from build123d import *

# Parameters (mm, degrees)
SKETCH1_R           = 2.2
SKETCH1_R_2         = 1.7
BOSS_EXTRUDE1_DEPTH = 6


with BuildPart() as part:
    # Sketch1 → Boss-Extrude1 (new body)
    with BuildSketch(Plane.XY.offset(3)):
        with BuildLine():
            Line((40.555136163, -29), (40.555136163, 17))
            ThreePointArc((40.555136163, 17), (42.019602257, 20.535533906), (45.555136163, 22))
            Line((45.555136163, 22), (54, 22))
            Line((54, 22), (74, 42))
            Line((74, 42), (74, 64))
            ThreePointArc((74, 64), (72.828427125, 66.828427125), (70, 68))
            Line((70, 68), (69, 68))
            ThreePointArc((69, 68), (68.292893219, 68.292893219), (68, 69))
            Line((68, 69), (68, 100))
            Line((68, 100), (56.5, 100))
            Line((56.5, 100), (56.5, 62.4))
            ThreePointArc((56.5, 62.4), (55.035533906, 58.864466094), (51.5, 57.4))
            Line((51.5, 57.4), (46.5, 57.4))
            ThreePointArc((46.5, 57.4), (42.964466094, 58.864466094), (41.5, 62.4))
            Line((41.5, 62.4), (41.5, 100))
            Line((41.5, 100), (-41.5, 100))
            Line((-41.5, 100), (-41.5, 62.4))
            ThreePointArc((-41.5, 62.4), (-42.964466094, 58.864466094), (-46.5, 57.4))
            Line((-46.5, 57.4), (-51.5, 57.4))
            ThreePointArc((-51.5, 57.4), (-55.035533906, 58.864466094), (-56.5, 62.4))
            Line((-56.5, 62.4), (-56.5, 100))
            Line((-56.5, 100), (-68, 100))
            Line((-68, 100), (-68, 69))
            ThreePointArc((-68, 69), (-68.292893219, 68.292893219), (-69, 68))
            Line((-69, 68), (-70, 68))
            ThreePointArc((-70, 68), (-72.828427125, 66.828427125), (-74, 64))
            Line((-74, 64), (-74, 42))
            Line((-74, 42), (-54, 22))
            Line((-54, 22), (-45.555136163, 22))
            ThreePointArc((-45.555136163, 22), (-42.019602257, 20.535533906), (-40.555136163, 17))
            Line((-40.555136163, 17), (-40.555136163, -29))
            ThreePointArc((-40.555136163, -29), (-42.019602257, -32.535533906), (-45.555136163, -34))
            Line((-45.555136163, -34), (-66, -34))
            Line((-66, -34), (-74, -42))
            Line((-74, -42), (-74, -64))
            ThreePointArc((-74, -64), (-72.828427125, -66.828427125), (-70, -68))
            Line((-70, -68), (-69, -68))
            ThreePointArc((-69, -68), (-68.292893219, -68.292893219), (-68, -69))
            Line((-68, -69), (-68, -100))
            Line((-68, -100), (-56.5, -100))
            Line((-56.5, -100), (-56.5, -61.8))
            ThreePointArc((-56.5, -61.8), (-55.035533906, -58.264466094), (-51.5, -56.8))
            Line((-51.5, -56.8), (-25.5, -56.8))
            ThreePointArc((-25.5, -56.8), (-21.964466094, -58.264466094), (-20.5, -61.8))
            Line((-20.5, -61.8), (-20.5, -100))
            Line((-20.5, -100), (20.5, -100))
            Line((20.5, -100), (20.5, -61.8))
            ThreePointArc((20.5, -61.8), (21.964466094, -58.264466094), (25.5, -56.8))
            Line((25.5, -56.8), (51.5, -56.8))
            ThreePointArc((51.5, -56.8), (55.035533906, -58.264466094), (56.5, -61.8))
            Line((56.5, -61.8), (56.5, -100))
            Line((56.5, -100), (68, -100))
            Line((68, -100), (68, -69))
            ThreePointArc((68, -69), (68.292893219, -68.292893219), (69, -68))
            Line((69, -68), (70, -68))
            ThreePointArc((70, -68), (72.828427125, -66.828427125), (74, -64))
            Line((74, -64), (74, -42))
            Line((74, -42), (66, -34))
            Line((66, -34), (45.555136163, -34))
            ThreePointArc((45.555136163, -34), (42.019602257, -32.535533906), (40.555136163, -29))
        make_face()
        with Locations(Location((-20, 19, 0), (0, 0, 180))):
            Circle(SKETCH1_R, mode=Mode.SUBTRACT)
        with Locations(Location((60, 49, 0), (0, 0, 180))):
            Circle(SKETCH1_R, mode=Mode.SUBTRACT)
        with Locations(Location((20, 49, 0), (0, 0, 180))):
            Circle(SKETCH1_R, mode=Mode.SUBTRACT)
        with Locations(Location((33.555136163, 4.3, 0), (0, 0, 180))):
            Circle(SKETCH1_R, mode=Mode.SUBTRACT)
        with Locations(Location((30, -17.1, 0), (0, 0, 180))):
            Circle(SKETCH1_R_2, mode=Mode.SUBTRACT)
        with Locations(Location((-33.555136163, 12.3, 0), (0, 0, 180))):
            Circle(SKETCH1_R, mode=Mode.SUBTRACT)
        with Locations(Location((-30, -34.1, 0), (0, 0, 180))):
            Circle(SKETCH1_R_2, mode=Mode.SUBTRACT)
        with Locations(Location((62, -72.2, 0), (0, 0, 180))):
            Circle(SKETCH1_R, mode=Mode.SUBTRACT)
        with Locations(Location((-62, -72.2, 0), (0, 0, 180))):
            Circle(SKETCH1_R, mode=Mode.SUBTRACT)
        with Locations(Location((-15, -72.2, 0), (0, 0, 180))):
            Circle(SKETCH1_R, mode=Mode.SUBTRACT)
        with Locations(Location((15, -72.2, 0), (0, 0, 180))):
            Circle(SKETCH1_R, mode=Mode.SUBTRACT)
        with Locations(Location((-30, -17.1, 0), (0, 0, 180))):
            Circle(SKETCH1_R_2, mode=Mode.SUBTRACT)
        with Locations(Location((-33.555136163, 4.3, 0), (0, 0, 180))):
            Circle(SKETCH1_R, mode=Mode.SUBTRACT)
        with Locations(Location((30, -34.1, 0), (0, 0, 180))):
            Circle(SKETCH1_R_2, mode=Mode.SUBTRACT)
        with Locations(Location((33.555136163, 12.3, 0), (0, 0, 180))):
            Circle(SKETCH1_R, mode=Mode.SUBTRACT)
        with Locations(Location((20, 19, 0), (0, 0, 180))):
            Circle(SKETCH1_R, mode=Mode.SUBTRACT)
        with Locations(Location((-20, 49, 0), (0, 0, 180))):
            Circle(SKETCH1_R, mode=Mode.SUBTRACT)
        with Locations(Location((-60, 49, 0), (0, 0, 180))):
            Circle(SKETCH1_R, mode=Mode.SUBTRACT)
        with BuildLine():
            Line((38.2, 95.1), (38.2, 93.1))
            ThreePointArc((38.2, 93.1), (36, 90.9), (33.8, 93.1))
            Line((33.8, 93.1), (33.8, 95.1))
            ThreePointArc((33.8, 95.1), (36, 97.3), (38.2, 95.1))
        make_face(mode=Mode.SUBTRACT)
        with BuildLine():
            Line((64.2, 72.1), (64.2, 70.1))
            ThreePointArc((64.2, 70.1), (62, 67.9), (59.8, 70.1))
            Line((59.8, 70.1), (59.8, 72.1))
            ThreePointArc((59.8, 72.1), (62, 74.3), (64.2, 72.1))
        make_face(mode=Mode.SUBTRACT)
        with BuildLine():
            Line((-38.2, 70.1), (-38.2, 72.1))
            ThreePointArc((-38.2, 72.1), (-36, 74.3), (-33.8, 72.1))
            Line((-33.8, 72.1), (-33.8, 70.1))
            ThreePointArc((-33.8, 70.1), (-36, 67.9), (-38.2, 70.1))
        make_face(mode=Mode.SUBTRACT)
        with BuildLine():
            Line((-64.2, 93.1), (-64.2, 95.1))
            ThreePointArc((-64.2, 95.1), (-62, 97.3), (-59.8, 95.1))
            Line((-59.8, 95.1), (-59.8, 93.1))
            ThreePointArc((-59.8, 93.1), (-62, 90.9), (-64.2, 93.1))
        make_face(mode=Mode.SUBTRACT)
        with BuildLine():
            Line((12.8, -94), (12.8, -92))
            ThreePointArc((12.8, -92), (15, -89.8), (17.2, -92))
            Line((17.2, -92), (17.2, -94))
            ThreePointArc((17.2, -94), (15, -96.2), (12.8, -94))
        make_face(mode=Mode.SUBTRACT)
        with BuildLine():
            Line((-12.8, -92), (-12.8, -94))
            ThreePointArc((-12.8, -94), (-15, -96.2), (-17.2, -94))
            Line((-17.2, -94), (-17.2, -92))
            ThreePointArc((-17.2, -92), (-15, -89.8), (-12.8, -92))
        make_face(mode=Mode.SUBTRACT)
        with BuildLine():
            Line((-59.8, -92), (-59.8, -94))
            ThreePointArc((-59.8, -94), (-62, -96.2), (-64.2, -94))
            Line((-64.2, -94), (-64.2, -92))
            ThreePointArc((-64.2, -92), (-62, -89.8), (-59.8, -92))
        make_face(mode=Mode.SUBTRACT)
        with BuildLine():
            Line((59.8, -94), (59.8, -92))
            ThreePointArc((59.8, -92), (62, -89.8), (64.2, -92))
            Line((64.2, -92), (64.2, -94))
            ThreePointArc((64.2, -94), (62, -96.2), (59.8, -94))
        make_face(mode=Mode.SUBTRACT)
        with BuildLine():
            Line((-64.2, 70.1), (-64.2, 72.1))
            ThreePointArc((-64.2, 72.1), (-62, 74.3), (-59.8, 72.1))
            Line((-59.8, 72.1), (-59.8, 70.1))
            ThreePointArc((-59.8, 70.1), (-62, 67.9), (-64.2, 70.1))
        make_face(mode=Mode.SUBTRACT)
        with BuildLine():
            Line((-38.2, 93.1), (-38.2, 95.1))
            ThreePointArc((-38.2, 95.1), (-36, 97.3), (-33.8, 95.1))
            Line((-33.8, 95.1), (-33.8, 93.1))
            ThreePointArc((-33.8, 93.1), (-36, 90.9), (-38.2, 93.1))
        make_face(mode=Mode.SUBTRACT)
        with BuildLine():
            Line((64.2, 95.1), (64.2, 93.1))
            ThreePointArc((64.2, 93.1), (62, 90.9), (59.8, 93.1))
            Line((59.8, 93.1), (59.8, 95.1))
            ThreePointArc((59.8, 95.1), (62, 97.3), (64.2, 95.1))
        make_face(mode=Mode.SUBTRACT)
        with BuildLine():
            Line((38.2, 72.1), (38.2, 70.1))
            ThreePointArc((38.2, 70.1), (36, 67.9), (33.8, 70.1))
            Line((33.8, 70.1), (33.8, 72.1))
            ThreePointArc((33.8, 72.1), (36, 74.3), (38.2, 72.1))
        make_face(mode=Mode.SUBTRACT)
    extrude(amount=-BOSS_EXTRUDE1_DEPTH)


solid = part.part
Geometry: final body of the model. Coordinates: model frame, mm. A direction names the side the tool comes from. Coordinates: 2 decimals unless noted, no trailing zeros. Loops run counter-clockwise (first coordinate to the right, second up) from the corner with the lowest first, then second, coordinate; pieces in that order, holes last. Notation, with made-up numbers: (27, -0.5) - (77, -0.5) arc R17 cw to (77, 12.5) - close; hole circle Ø11 at (26.5, 52.25). An arc over 180 degrees is marked (long way). Put each result on its own line as item: value. Start each with the question number.
Q1. Cut plane D-D, the plane z = 0.15. Give the number of separate pieces and of enclosed holes in the cut face, and give its area (3 significant figures).
Q2. Cut plane C-C, the plane y = 12.3. Return loops of the section in (x, z), and give its area (3 significant figures).
Q3. Set-up query: faces 4 (the cylindrical face through (-62, -96.2, 0)), 5 (the flat face through (-70, -38, 0)), 6 (the cylindrical face through (55, -58.23, 0.04)). Return all of +Z, -Z, +X, -X, +Y, -Y with unobstructed straight access to the full face (end or side cutting, diameter ignored); none if empty.
Q4. Pin query (flat end, axial travel): pin 1 Ø0.8 at (x, z) = (-69.5, -0.5) entering from +Y; pin 2 Ø2 at (y, z) = (94, 1.5) entering from -X; pin 3 Ø0.6 at (y, z) = (71, -0.5) entering from +X. Return the tip coordinate at first contact, or that it passes through.
Q5. Cut plane B-B, the plane x = 15. Return loops of the section in (y, z), and give its area (3 significant figures).
Q6. Pull-direction query (X, two-part tool) for faces 1 (the cylindrical face through (15, -96.2, 0)), 2 (the flat face through (56, -34, 0)), 3 (the flat face through (74, -53, 0)); classes: released by +X, released by -X, zero draft, split by the parting line, or undercut.
Q7. Cut plane A-A, the plane y = -72.2. Return loops of the section in (x, z), and give its area (3 significant figures).
Q8. Line query: line 1 (X direction, y = -88.5, z = 0.3); line 2 (Y direction, x = -30, z = -0.1); line 3 (X direction, y = 4, z = 0.8). Output: solid intervals per line, ascending.
Filled sheet:
1. separate pieces: 1
1. enclosed holes: 30
1. area: 19,700 mm²
2. outline: (-40.56, -3) - (-35.76, -3) - (-35.76, 3) - (-40.56, 3) - close; (-31.36, -3) - (31.36, -3) - (31.36, 3) - (-31.36, 3) - close; (35.76, -3) - (40.56, -3) - (40.56, 3) - (35.76, 3) - close
2. area: 434 mm²
3. face 4: +Z, -Z
3. face 5: +Z, -Z, -X
3. face 6: +Z, -Z, -Y
4. pin 1: y = 68
4. pin 2: x = -68
4. pin 3: x = 68
5. outline: (-100, -3) - (-96.2, -3) - (-96.2, 3) - (-100, 3) - close; (-89.8, -3) - (-74.4, -3) - (-74.4, 3) - (-89.8, 3) - close; (-70, -3) - (100, -3) - (100, 3) - (-70, 3) - close
5. area: 1,140 mm²
6. face 1: undercut
6. face 2: zero draft
6. face 3: released by +X
7. outline: (-68, -3) - (-64.2, -3) - (-64.2, 3) - (-68, 3) - close; (-59.8, -3) - (-56.5, -3) - (-56.5, 3) - (-59.8, 3) - close; (-20.5, -3) - (-17.2, -3) - (-17.2, 3) - (-20.5, 3) - close; (-12.8, -3) - (12.8, -3) - (12.8, 3) - (-12.8, 3) - close; (17.2, -3) - (20.5, -3) - (20.5, 3) - (17.2, 3) - close; (56.5, -3) - (59.8, -3) - (59.8, 3) - (56.5, 3) - close; (64.2, -3) - (68, -3) - (68, 3) - (64.2, 3) - close
7. area: 278 mm²
8. line 1: -68 to -56.5, -20.5 to 20.5, 56.5 to 68
8. line 2: -56.8 to -35.8, -32.4 to -18.8, -15.4 to 100
8. line 3: -40.56 to -35.73, -31.38 to 31.38, 35.73 to 40.56
